Part print with two shaded views. Sizes in mm from the minimum x, y, z corner. Round coordinates to 2 decimals unless told otherwise and drop trailing zeros. Order: outer loops, then holes, each group sorted by start corner. A loop starts at its lowest first (then second) coordinate and runs counter-clockwise, first axis right, second up. Notation, with made-up numbers: (-9, -4.75) -> (41, -4.75) arc R27 cw to (41, 18.25) -> close; hole circle Ø11 at (29, 1.5). An arc over 180 degrees is marked (long way). Put each result on its own line as item: value. Start each with the question number.
Q1. Pull direction X, two halves, no side cores. Call the marked faces 1, 2 and 3: released by +X, released by -X, zero draft, split by the parting line, or undercut.
Q2. Cut at B-B, the plane y = 15.5. List the corners of the cut face in (x, z), and give its area (4 significant figures).
Q3. Cut at D-D, the plane z = 4.5. List the corners of the cut face in (x, y).
Q4. Probe L1, parallel to X at y = 19, z = 3; L2, parallel to X at y = 15.5, z = 3.25; L3, parallel to Z at x = 8.5, y = 28.5. List the from-to ranges inside material, lowest first.
Q5. Flat gauge pins, fed straight in: P1, Ø1, axis at x = 11, y = 30, coming from the +Z side; P2, Ø1, axis at y = 29, z = 2, coming from the -X side; P3, Ø4, axis at x = 33.5, y = 18.5, coming from the +Z side. Where does each tip first touch, or does it go through?
Q6. Cut at C-C, the plane z = 2. List the corners of the cut face in (x, y), and give its area (3 significant figures).
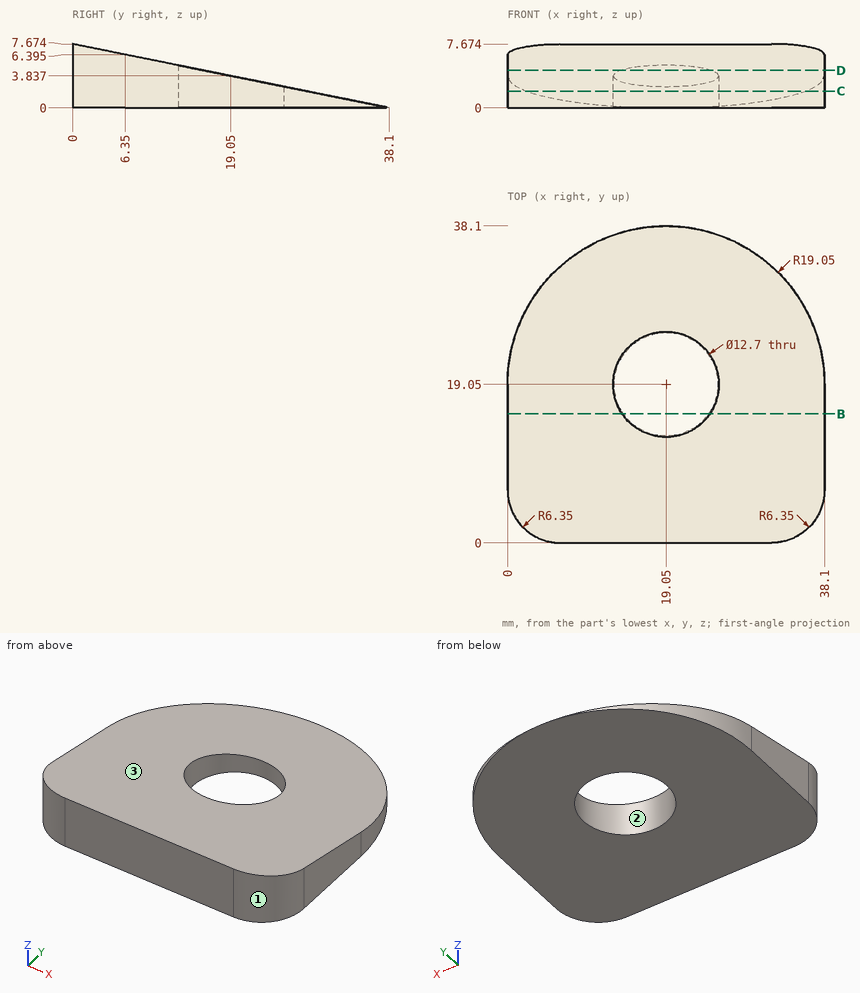
Ans:
1. face 1: released by +X
1. face 2: undercut
1. face 3: zero draft
2. outline: (0, 0) -> (13.79, 0) -> (13.79, 4.55) -> (0, 4.55) -> close; (24.31, 0) -> (38.1, 0) -> (38.1, 4.55) -> (24.31, 4.55) -> close
2. area: 125.5 mm^2
3. outline: (0, 6.35) arc R6.35 ccw to (6.35, 0) -> (31.75, 0) arc R6.35 ccw to (38.1, 6.35) -> (38.1, 15.76) -> (24.48, 15.76) arc R6.35 cw to (13.62, 15.76) -> (0, 15.76) -> close
4. L1: x = 0 to 12.7, 25.4 to 38.1
4. L2: x = 0 to 13.79, 24.31 to 38.1
4. L3: z = 0 to 1.93
5. P1: stops at z = 1.73
5. P2: stops at x = 2.51
5. P3: stops at z = 4.35
6. outline: (0, 6.35) arc R6.35 ccw to (6.35, 0) -> (31.75, 0) arc R6.35 ccw to (38.1, 6.35) -> (38.1, 19.05) arc R19.05 ccw to (35.77, 28.17) -> (2.33, 28.17) arc R19.05 ccw to (0, 19.05) -> close; hole circle Ø12.7 at (19.05, 19.05)
6. area: 916 mm^2
